Part model, mm, in its own coordinate system. A direction names the side the tool comes from. Give positions to 0.01 mm unless a question says otherwise; leave off trailing zeros. Order: outer loops, then holes, each group sorted by start corner. A loop starts at its lowest first (then second) coordinate and runs counter-clockwise, first axis right, second up. Notation, with made-up numbers: (66, 5) - (77, 5) arc R15 cw to (77, 11) - close; hole circle Ø6 at (30, -25.5). An arc over 180 degrees is marked (long way). One line per item, written item: value.
```python
from build123d import *

# Parameters (mm, degrees)
SKETCH1_W                    = 100
SKETCH1_H                    = 50
BASE_FLANGE1_DEPTH           = 3
SKETCH2_R                    = 11.05
SKETCH2_R_2                  = 1.75
CUT_EXTRUDE1_DEPTH           = 104.121287812
SKETCH3_R                    = 1.75
CUT_EXTRUDE2_DEPTH           = 104.121287812
CIRPATTERN1_COUNT            = 4
CUT_EXTRUDE3_DEPTH           = 104.121287812
SKETCHED_BEND2_OUTLINE_W     = 3
SKETCHED_BEND2_OUTLINE_H     = 50
SKETCHED_BEND2_DEPTH         = 47.020021532
SKETCHED_START               = 47.383443248
SKETCHED_BEND2_2_OUTLINE_W   = 47.979978468
SKETCHED_BEND2_2_OUTLINE_H   = 50
SKETCHED_BEND2_2_OUTLINE_R   = 1.75
SKETCHED_BEND2_2_OUTLINE_R_2 = 11.05
SKETCHED_BEND2_2_DEPTH       = 2.636578284
SKETCHED_START_2             = 47.020021532
SKETCHED_BEND2_3_OUTLINE_W   = 47.979978468
SKETCHED_BEND2_3_OUTLINE_H   = 50
SKETCHED_BEND2_3_OUTLINE_R   = 1.75
SKETCHED_BEND2_3_OUTLINE_R_2 = 11.05
SKETCHED_BEND2_3_DEPTH       = 3.7366
SKETCHED_START_3             = -26
SKETCHED_BEND2_4_DEPTH       = 52
BOSS_EXTRUDE1_DEPTH          = 3
CHAMFER1_SIZE                = 5
CHAMFER2_SIZE                = 0.3
CHAMFER3_SIZE                = 0.3


with BuildPart() as part:
    # Base-Flange1: sheet metal written as solids
    # Sketch1 → Base-Flange1 (new body)
    with BuildSketch(Plane(origin=(0, 0, 0), x_dir=(1, 0, 0), z_dir=(0, 1, 0))):
        with Locations((50, 0)):
            Rectangle(SKETCH1_W, SKETCH1_H)
    extrude(amount=-BASE_FLANGE1_DEPTH)

    # Sketch2 → Cut-Extrude1 (cut, through all)
    with BuildSketch(Plane(origin=(0, 0, 0), x_dir=(1, 0, 0), z_dir=(0, 1, 0))):
        with Locations(Location((21, 0, 0), (0, 0, 270))):
            Circle(SKETCH2_R)
        with Locations(Location((5.5, 15.5, 0), (0, 0, 270))):
            Circle(SKETCH2_R_2)
        with Locations(Location((36.5, 15.5, 0), (0, 0, 270))):
            Circle(SKETCH2_R_2)
        with Locations(Location((36.5, -15.5, 0), (0, 0, 270))):
            Circle(SKETCH2_R_2)
        with Locations(Location((5.5, -15.5, 0), (0, 0, 270))):
            Circle(SKETCH2_R_2)
    extrude(amount=-CUT_EXTRUDE1_DEPTH, mode=Mode.SUBTRACT)

    # Sketch3 → Cut-Extrude2 (cut, through all)
    with BuildSketch(Plane(origin=(0, 0, 0), x_dir=(1, 0, 0), z_dir=(0, 1, 0))):
        with Locations(Location((11.100505063, 9.899494937, 0), (0, 0, 270))):
            Circle(SKETCH3_R)
    cut_extrude2 = extrude(amount=-CUT_EXTRUDE2_DEPTH, mode=Mode.SUBTRACT)

    # CirPattern1: Cut-Extrude2 ×4 about axis
    cirpattern1_axis = Axis((21, 0, 0), (0, 1, 0))
    for i in range(1, CIRPATTERN1_COUNT):
        add(cut_extrude2.rotate(cirpattern1_axis, i * 360 / CIRPATTERN1_COUNT), mode=Mode.SUBTRACT)

    # Sketch4 → Cut-Extrude3 (cut, through all)
    with BuildSketch(Plane(origin=(0, 0, 0), x_dir=(1, 0, 0), z_dir=(0, 1, 0))):
        with BuildLine():
            Line((59, 17.1), (89, 17.1))
            ThreePointArc((89, 17.1), (91.1, 15), (89, 12.9))
            Line((89, 12.9), (59, 12.9))
            ThreePointArc((59, 12.9), (56.9, 15), (59, 17.1))
        make_face()
        with BuildLine():
            Line((59, -12.9), (89, -12.9))
            ThreePointArc((89, -12.9), (91.1, -15), (89, -17.1))
            Line((89, -17.1), (59, -17.1))
            ThreePointArc((59, -17.1), (56.9, -15), (59, -12.9))
        make_face()
    extrude(amount=-CUT_EXTRUDE3_DEPTH, mode=Mode.SUBTRACT)

    # Sketched Bend2: read off the stored shape, not the designer's step
    # Sketched Bend2 outline → Sketched Bend2 (cut)
    with BuildSketch(Plane.YZ):
        with Locations((-1.5, 0)):
            Rectangle(SKETCHED_BEND2_OUTLINE_W, SKETCHED_BEND2_OUTLINE_H)
    extrude(amount=SKETCHED_BEND2_DEPTH, mode=Mode.SUBTRACT)

    # Sketched Bend2 2 outline → Sketched Bend2 2 (add)
    with BuildSketch(Plane.YZ.offset(SKETCHED_START)):
        with Locations((23.989989234, 0)):
            Rectangle(SKETCHED_BEND2_2_OUTLINE_W, SKETCHED_BEND2_2_OUTLINE_H)
        with Locations((11.479978468, -15.5)):
            Circle(SKETCHED_BEND2_2_OUTLINE_R, mode=Mode.SUBTRACT)
        with Locations((17.080483531, -9.899494937)):
            Circle(SKETCHED_BEND2_2_OUTLINE_R, mode=Mode.SUBTRACT)
        with Locations((42.479978468, -15.5)):
            Circle(SKETCHED_BEND2_2_OUTLINE_R, mode=Mode.SUBTRACT)
        with Locations((36.879473404, -9.899494937)):
            Circle(SKETCHED_BEND2_2_OUTLINE_R, mode=Mode.SUBTRACT)
        with Locations((17.080483531, 9.899494937)):
            Circle(SKETCHED_BEND2_2_OUTLINE_R, mode=Mode.SUBTRACT)
        with Locations((11.479978468, 15.5)):
            Circle(SKETCHED_BEND2_2_OUTLINE_R, mode=Mode.SUBTRACT)
        with Locations((26.979978468, 0)):
            Circle(SKETCHED_BEND2_2_OUTLINE_R_2, mode=Mode.SUBTRACT)
        with Locations((36.879473404, 9.899494937)):
            Circle(SKETCHED_BEND2_2_OUTLINE_R, mode=Mode.SUBTRACT)
        with Locations((42.479978468, 15.5)):
            Circle(SKETCHED_BEND2_2_OUTLINE_R, mode=Mode.SUBTRACT)
    extrude(amount=SKETCHED_BEND2_2_DEPTH)

    # Sketched Bend2 3 outline → Sketched Bend2 3 (add)
    with BuildSketch(Plane.YZ.offset(SKETCHED_START_2)):
        with Locations((23.989989234, 0)):
            Rectangle(SKETCHED_BEND2_3_OUTLINE_W, SKETCHED_BEND2_3_OUTLINE_H)
        with Locations((11.479978468, -15.5)):
            Circle(SKETCHED_BEND2_3_OUTLINE_R, mode=Mode.SUBTRACT)
        with Locations((17.080483531, -9.899494937)):
            Circle(SKETCHED_BEND2_3_OUTLINE_R, mode=Mode.SUBTRACT)
        with Locations((42.479978468, -15.5)):
            Circle(SKETCHED_BEND2_3_OUTLINE_R, mode=Mode.SUBTRACT)
        with Locations((36.879473404, -9.899494937)):
            Circle(SKETCHED_BEND2_3_OUTLINE_R, mode=Mode.SUBTRACT)
        with Locations((17.080483531, 9.899494937)):
            Circle(SKETCHED_BEND2_3_OUTLINE_R, mode=Mode.SUBTRACT)
        with Locations((11.479978468, 15.5)):
            Circle(SKETCHED_BEND2_3_OUTLINE_R, mode=Mode.SUBTRACT)
        with Locations((26.979978468, 0)):
            Circle(SKETCHED_BEND2_3_OUTLINE_R_2, mode=Mode.SUBTRACT)
        with Locations((36.879473404, 9.899494937)):
            Circle(SKETCHED_BEND2_3_OUTLINE_R, mode=Mode.SUBTRACT)
        with Locations((42.479978468, 15.5)):
            Circle(SKETCHED_BEND2_3_OUTLINE_R, mode=Mode.SUBTRACT)
    extrude(amount=SKETCHED_BEND2_3_DEPTH)

    # Sketched Bend2 4 outline → Sketched Bend2 4 (cut)
    with BuildSketch(Plane.XY.offset(SKETCHED_START_3)):
        with BuildLine():
            Line((50.756621532, 47.979978468), (50.020021532, 47.979978468))
            Line((50.020021532, 47.979978468), (50.020021532, 0.7366))
            ThreePointArc((50.020021532, 0.7366), (50.235766677, 0.215745145), (50.756621532, 0))
            Line((50.756621532, 0), (50.756621532, 47.979978468))
        make_face()
        with BuildLine():
            ThreePointArc((50.756621532, -3), (48.114446333, -1.905575198), (47.020021532, 0.7366))
            Line((47.020021532, 0.7366), (47.020021532, -3))
            Line((47.020021532, -3), (50.756621532, -3))
        make_face()
    extrude(amount=SKETCHED_BEND2_4_DEPTH, mode=Mode.SUBTRACT)

    # Sketch6 → Boss-Extrude1 (add)
    with BuildSketch(Plane.XY.offset(25)):
        Polygon((50.020021532, 20), (63.020021532, 0), (52.020021532, 0), (50.020021532, 3.076923077), align=None)
    boss_extrude1 = extrude(amount=-BOSS_EXTRUDE1_DEPTH)

    # Mirror1: Boss-Extrude1 across plane
    add(boss_extrude1.mirror(Plane.XY))

    # Chamfer1
    chamfer1_edges = [part.edges().sort_by_distance(p)[0] for p in [
        (100, -1.5, -25),
        (100, -1.5, 25),
        (48.520021532, 47.979978468, -25),
        (48.520021532, 47.979978468, 25),
    ]]
    chamfer(chamfer1_edges, length=CHAMFER1_SIZE)

    # Chamfer2
    chamfer2_edges = [part.edges().sort_by_distance(p)[0] for p in [
        (74, 0, -17.1),
        (91.1, 0, -15),
        (74, 0, -12.9),
        (56.9, 0, -15),
        (74, 0, 12.9),
        (91.1, 0, 15),
        (74, 0, 17.1),
        (56.9, 0, 15),
        (56.9, -3, 15),
        (74, -3, 17.1),
        (91.1, -3, 15),
        (74, -3, 12.9),
        (56.9, -3, -15),
        (74, -3, -12.9),
        (91.1, -3, -15),
        (74, -3, -17.1),
        (47.020021532, 15.929978468, 0),
        (50.020021532, 15.929978468, 0),
        (47.020021532, 40.729978468, -15.5),
        (50.020021532, 40.729978468, -15.5),
        (47.020021532, 9.729978468, -15.5),
        (50.020021532, 9.729978468, -15.5),
        (47.020021532, 9.729978468, 15.5),
        (50.020021532, 9.729978468, 15.5),
        (47.020021532, 40.729978468, 15.5),
        (50.020021532, 40.729978468, 15.5),
    ]]
    chamfer(chamfer2_edges, length=CHAMFER2_SIZE)

    # Chamfer3
    chamfer3_edges = [part.edges().sort_by_distance(p)[0] for p in [
        (47.020021532, 35.129473404, -9.899494937),
        (50.020021532, 35.129473404, -9.899494937),
        (47.020021532, 35.129473404, 9.899494937),
        (50.020021532, 35.129473404, 9.899494937),
        (47.020021532, 15.330483531, 9.899494937),
        (50.020021532, 15.330483531, 9.899494937),
        (47.020021532, 15.330483531, -9.899494937),
        (50.020021532, 15.330483531, -9.899494937),
    ]]
    chamfer(chamfer3_edges, length=CHAMFER3_SIZE)


solid = part.part
```
1) Slice it at D-D on x = 54. Write the cut outline in (y, z), then the cut area to 3 significant figures.
Answer:
outline: (-3, -25) - (13.88, -25) - (13.88, -22) - (0, -22) - (0, 22) - (13.88, 22) - (13.88, 25) - (-3, 25) - close
area: 233 mm2
2) Two-plate mould, pull along Z, no slides. Class faces 1 (the face through (58, 6, 25)), 2 (the face through (48.503, 43.421, -14.024)), 3 (the face through (58, 6, -25)): pulls with the +Z half, pulls with the -Z half, needs draft (parallel to the pull), parting line crosses it, or undercut.
Answer:
face 1: pulls with the +Z half
face 2: undercut
face 3: pulls with the -Z half
3) Drop flat-ended pins along their axis: P1, Ø5.5, axis at y = 36.88, z = 9.9, coming from the +X side; P2, Ø12, axis at x = 85, z = 4.5, coming from the +Y side; P3, Ø3, axis at y = 36.88, z = -9.9, coming from the -X side. Give the stop position or say it passes through.
Answer:
P1: stops at x = 50.02
P2: stops at y = 0
P3: passes through
4) Wall check: line 1 along Y through (x, z) = (48.7, 15.5); line 2 along Z through (x, y) = (52, 8); line 3 along Y through (x, z) = (85.5, 8.5). Give the ranges that are in metal, low to high. Write a range as [from, to].
Answer:
line 1: y = [-2.38, 9.73], [13.23, 40.73], [44.23, 47.98]
line 2: z = [-25, -22], [22, 25]
line 3: y = [-3, 0]
5) Slice it at C-C on z = -19. Write the cut outline in (x, y).
Answer:
outline: (47.02, 0.74) arc R3.74 ccw to (50.76, -3) - (100, -3) - (100, 0) - (50.76, 0) arc R0.74 cw to (50.02, 0.74) - (50.02, 47.98) - (47.02, 47.98) - close
6) Which spindle directions (+Z, -Z, +X, -X, +Y, -Y) get a long thin tool onto all of the face, cutting with end or side? Do faces 4 (the face through (48.5, 37.52, 3.32)), 5 (the face through (56.9, -1.5, 15)), 6 (the face through (56.79, -2.81, -15.05)), 7 (the face through (91.21, -0.19, -15.05)). Say none if no direction does.
Answer:
face 4: +X, -X
face 5: +Y, -Y
face 6: -Y
face 7: +Y
7) Slice it at B-B on x = 74.5. Write the cut outline in (y, z), then the cut area to 3 significant figures.
Answer:
outline: (-3, -25) - (0, -25) - (0, -17.4) - (-0.3, -17.1) - (-2.7, -17.1) - (-3, -17.4) - close; (-3, -12.6) - (-2.7, -12.9) - (-0.3, -12.9) - (0, -12.6) - (0, 12.6) - (-0.3, 12.9) - (-2.7, 12.9) - (-3, 12.6) - close; (-3, 17.4) - (-2.7, 17.1) - (-0.3, 17.1) - (0, 17.4) - (0, 25) - (-3, 25) - close
area: 124 mm2
8) Slice it at A-A on z = 0. Write the cut outline in (x, y), then the cut area to 3 significant figures.
Answer:
outline: (47.02, 0.74) arc R3.74 ccw to (50.76, -3) - (100, -3) - (100, 0) - (50.76, 0) arc R0.74 cw to (50.02, 0.74) - (50.02, 15.63) - (49.72, 15.93) - (47.32, 15.93) - (47.02, 15.63) - close; (47.02, 38.33) - (47.32, 38.03) - (49.72, 38.03) - (50.02, 38.33) - (50.02, 47.98) - (47.02, 47.98) - close
area: 234 mm2
